Can you work these out from the model? Positions are in its coordinate system, mm. A direction names the side the tool comes from. Coordinates: 2 decimals unless noted, no trailing zeros. Loops run counter-clockwise (first coordinate to the right, second up) from the corner with the lowest first, then second, coordinate; pieces in that order, holes last.
```python
from build123d import *

# Parameters (mm, degrees)
SKETCH1_8_W         = 203.2
SKETCH1_8_H         = 15.24
SKETCH1_8_W_2       = 50.8
SKETCH1_8_H_2       = 5.08
BOSS_EXTRUDE1_DEPTH = 3.429
SKETCH1_9_W         = 15.24
SKETCH1_9_H         = 35.56
BOSS_EXTRUDE2_DEPTH = 2.286
BOSS_EXTRUDE3_DEPTH = 3.81


# Read off the part's stored shape, not the designer's step: Revolve-Thin2
with BuildPart() as part:
    # Revolve-Thin2 outline → Revolve-Thin2 (revolve)
    with BuildSketch(Plane(origin=(-63.5, 0, 0), x_dir=(1, 0, 0), z_dir=(0, 0, 1))):
        Polygon((0, 152.4), (0, 0), (10.401925271, 0), (5.08, 152.4), align=None)
        Polygon((2.54, 2.54), (2.54, 149.86), (2.627150512, 149.86), (7.771678274, 2.54), align=None, mode=Mode.SUBTRACT)
    revolve(axis=Axis((-63.5, 0, 0), (0, 1, 0)))



with BuildPart() as body_2:
    # Sketch1<4> → Revolve1 (revolve)
    with BuildSketch(Plane.XY):
        Polygon((53.098074729, 0), (63.5, 0), (63.5, 152.4), (58.42, 152.4), align=None)
    revolve(axis=Axis((63.5, 0, 0), (0, 1, 0)))


with BuildPart() as body_3:
    # Sketch1<8> → Boss-Extrude1 (new, symmetric)
    with BuildSketch(Plane.XY):
        with Locations((0, 109.22)):
            Rectangle(SKETCH1_8_W, SKETCH1_8_H)
        with Locations((63.5, 119.38)):
            Rectangle(SKETCH1_8_W_2, SKETCH1_8_H_2)
        with Locations((-63.5, 119.38)):
            Rectangle(SKETCH1_8_W_2, SKETCH1_8_H_2)
    extrude(amount=BOSS_EXTRUDE1_DEPTH, both=True)

    # Sketch1<9> → Boss-Extrude2 (add, symmetric)
    with BuildSketch(Plane.XY):
        with Locations((0, 134.62)):
            Rectangle(SKETCH1_9_W, SKETCH1_9_H)
    extrude(amount=BOSS_EXTRUDE2_DEPTH, both=True)


with BuildPart() as part_1:
    add(part.part)

    add(body_2.part)  # Boss-Extrude3 merges body 2

    add(body_3.part)  # Boss-Extrude3 merges body 3
    # Sketch3 → Boss-Extrude3 (add, symmetric)
    with BuildSketch(Plane.XY):
        with BuildLine():
            Line((-101.6, 152.4), (101.6, 152.4))
            Line((101.6, 152.4), (111.76, 174.188190312))
            ThreePointArc((111.76, 174.188190312), (0, 166.616423921), (-111.76, 174.188190312))
            Line((-111.76, 174.188190312), (-101.6, 152.4))
        make_face()
    extrude(amount=BOSS_EXTRUDE3_DEPTH, both=True)


solid = part_1.part
```
Item 1: We'd pull the mould along X, two halves only. Please class faces 6 (the face through (85, 112, 3.429)), 7 (the face through (101.6, 109, 0)), 8 (the face through (-66.038, 136.086, -0.112)): +X half, -X half, draft (parallel to the pull), parting line (faces both ways), or undercut.
Results are:
face 6: draft
face 7: +X half
face 8: undercut
Item 2: Suppose I cut it at C-C, the plane x = 35. Please give me the cut outline in (y, z).
Results are:
outline: (101.6, -3.43) - (116.84, -3.43) - (116.84, 3.43) - (101.6, 3.43) - close; (152.4, -3.81) - (167.36, -3.81) - (167.36, 3.81) - (152.4, 3.81) - close
Item 3: Suppose I cut it at B-B, the plane y = 77.5. Please give me the cut outline in (x, z).
Results are:
outline: circle Ø15.39 at (-63.5, 0); circle Ø5.08 at (-63.5, 0); circle Ø15.39 at (63.5, 0); hole circle Ø10.31 at (-63.5, 0)
Item 4: I need wall thicknesses on line 1 along X through (y, z) = (81, -1.5); line 2 along X through (y, z) = (83.5, -2.25); line 3 along Y through (x, z) = (-3, 3.75). Which ranges of each line are inside material? Lowest first, please.
Results are:
line 1: x = -70.92 to -68.3, -65.55 to -61.45, -58.7 to -56.08, 56.08 to 70.92
line 2: x = -70.64 to -67.9, -64.68 to -62.32, -59.1 to -56.36, 56.36 to 70.64
line 3: y = 152.4 to 166.62
Item 5: On a 3-axis mill with a long thin cutter (end or side, diameter ignored), from which of +Z, -Z, +X, -X, +Y, -Y can I reach the whole of each face in a straight line? I mean faces 1 (the face through (88.9, 119, 0)), 2 (the face through (85, 112, -3.429)), 3 (the face through (-71.196, 77.267, -0.339)), 4 (the face through (7.62, 134, 0)), 5 (the face through (-88.9, 119, 0)). Say none if no direction works.
Results are:
face 1: +Z, -Z, +X
face 2: -Z, +X
face 3: none
face 4: +Z, -Z
face 5: +Z, -Z, -X
Item 6: I'm going to push flat-ended pins straight in: P1, Ø6, axis at x = -63, y = 115.5, coming from the -Z side; P2, Ø2, axis at y = 109, z = 0, coming from the +X side; P3, Ø12, axis at x = -2.5, y = 141, coming from the -Z side; P4, Ø3, axis at x = 53, z = 1.5, coming from the -Y side. Where does each tip first touch, or does it pass through?
Results are:
P1: stops at z = -6.47
P2: stops at x = 101.6
P3: stops at z = -2.29
P4: stops at y = 0
Item 7: Suppose I cut it at A-A, the plane x = -92. Please give me the cut outline in (y, z), plus the area to 3 significant figures.
Results are:
outline: (101.6, -3.43) - (116.84, -3.43) - (116.84, 3.43) - (101.6, 3.43) - close; (152.4, -3.81) - (171.74, -3.81) - (171.74, 3.81) - (152.4, 3.81) - close
area: 252 mm2
Item 8: Suppose I cut it at D-D, the plane x = 63.5. Please give me the cut outline in (y, z), plus the area to 3 significant figures.
Results are:
outline: (0, -10.4) - (152.4, -5.08) - (152.4, -3.81) - (169.05, -3.81) - (169.05, 3.81) - (152.4, 3.81) - (152.4, 5.08) - (0, 10.4) - close
area: 2,490 mm2
